Input: part model. Units: mm. Frame: model coordinates. A direction names the side the tool comes from. Coordinates: 2 decimals unless noted, no trailing zeros. Loops run counter-clockwise (first coordinate to the right, second up) from the corner with the lowest first, then second, coordinate; pieces in that order, holes last.
(1) Line query: L1, parallel to X at y = 2, z = -6.35; L2, parallel to Z at x = 1.5, y = 22; L3, parallel to Y at x = -1.75, z = 23. Output: solid intervals per line, ascending.
(2) Set-up query: faces 5 (the face through (-5.4, 6.35, -9.1)), 6 (the face through (-5.863, 30.275, 6.439)), 7 (the face through (-3, 3, -12.7)), 8 (the face through (-3, 16, 12.7)), 9 (the face through (-7.55, 14.9, 6.44)). Return all of +Z, -Z, +X, -X, +Y, -Y with unobstructed straight access to the full face (end or side cutting, diameter ignored); none if empty.
(3) Contact query for flat-ended pins moving along their axis: P1, Ø5.5, axis at x = -3.175, z = -6.35, coming from the +Y side; P2, Ø5, axis at x = 4, y = 19.5, coming from the +Z side; P3, Ø10, axis at x = -8, z = 11, coming from the +Y side; P4, Ø6.5, axis at x = -1, z = -9.5, coming from the +Y side. Output: stop coordinate, or through.
(4) Mould query, pull axis X, two halves, no side actions, for faces 1 (the face through (-0.147, 3.219, 18.096)), 2 (the face through (-1.521, 31.094, 6.13)), 3 (the face through (-3, 0, 7)), 4 (the face through (-12.7, 5, 7)). Classes: released by +X, released by -X, zero draft, split by the parting line, or undercut.
(5) Section D-D, the plane y = 15. Return loops of the section in (x, z), then the cut area to 3 significant figures.
(6) Section C-C, the plane y = 8. Return loops of the section in (x, z), then the cut area to 3 significant figures.
(7) Section B-B, the plane z = 12. Return loops of the section in (x, y).
(8) Section A-A, the plane z = -6.35. Return loops of the section in (x, y), then the cut area to 3 significant figures.
```python
from build123d import *

# Parameters (mm, degrees)
BOSS_EXTRUDE1_DEPTH = 12.7
CUT_EXTRUDE3_REACH  = 25.694
SKETCH2_R           = 4
SKETCH4_R           = 5
SKETCH4_R_2         = 4
BOSS_EXTRUDE2_DEPTH = 2
CUT_EXTRUDE4_REACH  = 14.7
SKETCH5_W           = 6.909894264
SKETCH5_H           = 12.7
SKETCH7_W           = 19.05
SKETCH7_H           = 6.35
BOSS_EXTRUDE3_DEPTH = 12.7
CUT_EXTRUDE5_DEPTH  = 12.7
SKETCH9_R           = 3.175
CUT_EXTRUDE6_DEPTH  = 12.7
SKETCH11_W          = 6.35
SKETCH11_H          = 14.564534892
CUT_EXTRUDE7_DEPTH  = 12.7


with BuildPart() as part:
    # Sketch1 → Boss-Extrude1 (new body)
    with BuildSketch(Plane.XY):
        Polygon((-12.7, 0), (12.7, 0), (12.7, 2.893589299), (-12.7, 49.577371669), align=None)
    extrude(amount=BOSS_EXTRUDE1_DEPTH)

    # Sketch2 → Cut-Extrude3 (cut, up to next)
    with BuildSketch(Plane(origin=(11.013915285, 5.992518901, 0), x_dir=(0.477925491, -0.878400379, 0), z_dir=(0.878400379, 0.477925491, 0)), mode=Mode.PRIVATE) as cut_extrude3_sk1:
        with Locations((-23.045255988, -6.35)):
            Circle(SKETCH2_R)
    cut_extrude3_tool1 = extrude(cut_extrude3_sk1.sketch, amount=-CUT_EXTRUDE3_REACH, mode=Mode.PRIVATE) & part.part
    add(cut_extrude3_tool1.solids().sort_by_distance((0, 26.23548, 6.35))[0], mode=Mode.SUBTRACT)

    # Sketch4 → Boss-Extrude2 (add)
    with BuildSketch(Plane(origin=(11.013915285, 5.992518901, 0), x_dir=(0.477925491, -0.878400379, 0), z_dir=(0.878400379, 0.477925491, 0))):
        with Locations((-23.045255988, -6.35)):
            Circle(SKETCH4_R)
        with Locations((-23.045255988, -6.35)):
            Circle(SKETCH4_R_2, mode=Mode.SUBTRACT)
    extrude(amount=BOSS_EXTRUDE2_DEPTH)

    # Sketch5 → Cut-Extrude4 (cut, up to next)
    with BuildSketch(Plane.XY.offset(12.7), mode=Mode.PRIVATE) as cut_extrude4_sk1:
        with Locations((-9.245052868, 43.227371669)):
            Rectangle(SKETCH5_W, SKETCH5_H)
    cut_extrude4_tool1 = extrude(cut_extrude4_sk1.sketch, amount=-CUT_EXTRUDE4_REACH, mode=Mode.PRIVATE) & part.part
    add(cut_extrude4_tool1.solids().sort_by_distance((-9.245053, 43.227372, 12.7))[0], mode=Mode.SUBTRACT)

    # Sketch7 → Boss-Extrude3 (add)
    with BuildSketch(Plane.XY.offset(12.7)):
        with Locations((-3.175, 3.175)):
            Rectangle(SKETCH7_W, SKETCH7_H)
    boss_extrude3 = extrude(amount=BOSS_EXTRUDE3_DEPTH)

    # Sketch8 → Cut-Extrude5 (cut)
    with BuildSketch(Plane.XY.offset(12.7)):
        Polygon((-8.612669272, 28.778496019), (-2.543015535, 17.622811212), (-12.7, 12.096536512), (-12.7, 26.554635929), align=None)
    extrude(amount=-CUT_EXTRUDE5_DEPTH, mode=Mode.SUBTRACT)

    # Sketch9 → Cut-Extrude6 (cut)
    with BuildSketch(Plane(origin=(0, 6.35, 0), x_dir=(1, 0, 0), z_dir=(0, 1, 0))):
        with Locations((-3.175, -19.05)):
            Circle(SKETCH9_R)
    cut_extrude6 = extrude(amount=-CUT_EXTRUDE6_DEPTH, mode=Mode.SUBTRACT)

    # Mirror1: Boss-Extrude3, Cut-Extrude6 across plane
    add(boss_extrude3.mirror(Plane.XY.offset(6.35)))
    add(cut_extrude6.mirror(Plane.XY.offset(6.35)), mode=Mode.SUBTRACT)

    # Sketch11 → Cut-Extrude7 (cut)
    with BuildSketch(Plane.XY.offset(12.7)):
        Polygon((-12.7, 26.554635929), (-3.034826868, 31.813322888), (-5.790105736, 36.877371669), (-12.7, 36.877371669), align=None)
        with Locations((9.525, 7.282267446)):
            Rectangle(SKETCH11_W, SKETCH11_H)
    extrude(amount=-CUT_EXTRUDE7_DEPTH, mode=Mode.SUBTRACT)


solid = part.part
```
Report:
1. L1: x = -12.7 to -6.35, 0 to 6.35
1. L2: z = 0 to 12.7
1. L3: y = 0 to 6.35
2. face 5: -Z, +X, -X, +Y
2. face 6: +Z, -Z, -X, +Y
2. face 7: -Z, +X, -X, +Y, -Y
2. face 8: +Z, +X, -X, +Y
2. face 9: +Z, -Z, -X
3. P1: passes through
3. P2: stops at z = 12.7
3. P3: stops at y = 31.81
3. P4: stops at y = 6.35
4. face 1: undercut
4. face 2: undercut
4. face 3: zero draft
4. face 4: released by -X
5. outline: (-7.36, 0) - (6.11, 0) - (6.11, 12.7) - (-7.36, 12.7) - close
5. area: 171 mm2
6. outline: (-12.7, 0) - (6.35, 0) - (6.35, 12.7) - (-12.7, 12.7) - close
6. area: 242 mm2
7. outline: (-12.7, 0) - (6.35, 0) - (6.35, 14.56) - (-3.03, 31.81) - (-8.61, 28.78) - (-2.54, 17.62) - (-12.7, 12.1) - close
8. outline: (-12.7, 0) - (-6.35, 0) - (-6.35, 6.35) - (-12.7, 6.35) - close; (0, 0) - (6.35, 0) - (6.35, 6.35) - (0, 6.35) - close
8. area: 80.6 mm2
